Design review of the part shown in the three views and the two pictorial views. Dimensions are in mm from the part's minimum x, y and z. Coordinates: 2 decimals unless noted, no trailing zeros. Loops run counter-clockwise (first coordinate to the right, second up) from the corner with the lowest first, then second, coordinate; pieces in that order, holes last. Notation, with made-up numbers: (26, 75.25) -> (50, 75.25) arc R22 cw to (50, 89.25) -> close; hole circle Ø9 at (-34, 84). An arc over 180 degrees is marked (long way). Use a Markdown table: item, result. Add a question column.
Q1. For probe 1 along Y at (x, z) = (13.5, 5.75) (3 decimals); probe 2 along Z at (x, y) = (6, 11); probe 3 along X at (y, z) = (10.25, 6.5), list the stretches that pass through material, from the lowest coordinate up.
Q2. Clearance check with flat-ended pins moving along their axes: pin 1 Ø4 at (x, z) = (19.5, 2) entering from +Y; pin 2 Ø1 at (y, z) = (20.5, 1) entering from -X; pin 3 Ø1.2 at (x, y) = (13, 12.5) entering from +Z. State where each tip first meets the part, or that it passes through.
Q3. Take a section at C-C on z = 5. Write out the cut boundary in (x, y) (3 decimals), plus the area to 3 significant figures.
Q4. Draft analysis for pull direction X (two halves, no side actions). For the marked faces 1, 2 and 3, state which applies: pulls with the +X half, pulls with the -X half, needs draft (parallel to the pull), parting line crosses it, or undercut.
Q5. Take a section at A-A on x = 13.5. Write out the cut boundary in (y, z) (3 decimals).
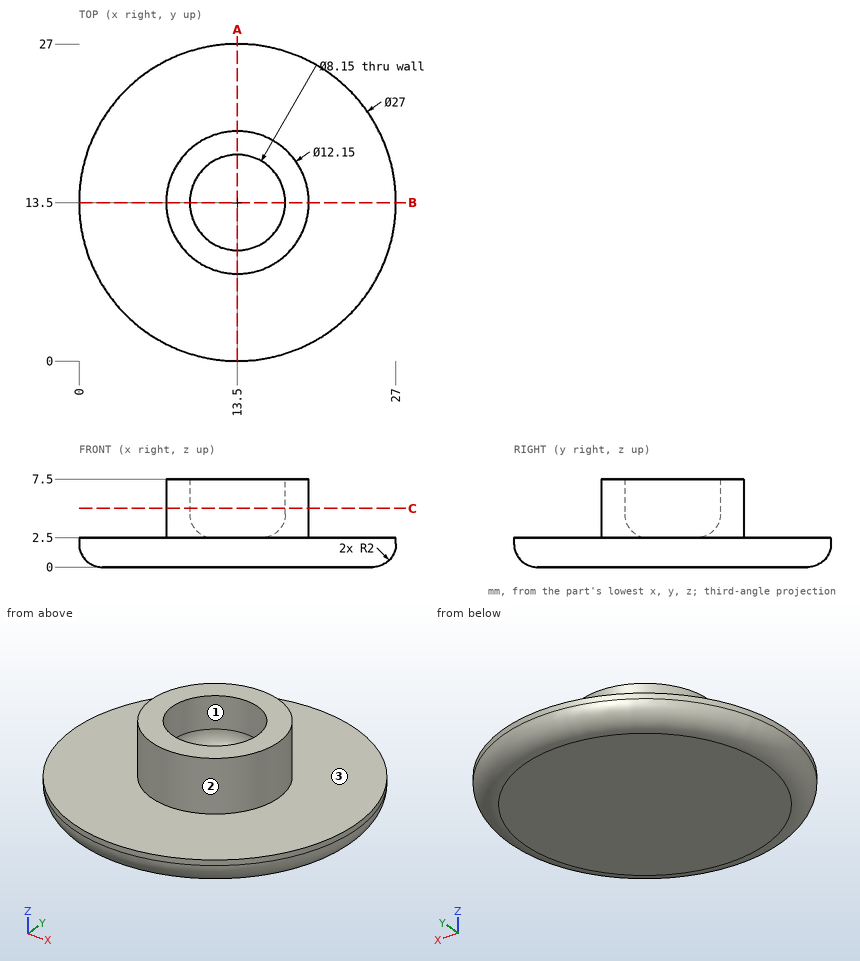
Answer list:
| question | item | result |
|---|---|---|
| 1 | probe 1 | 7.425 to 9.425, 17.575 to 19.575 |
| 1 | probe 2 | 0 to 2.5 |
| 1 | probe 3 | 8.37 to 11.04, 15.96 to 18.63 |
| 2 | pin 1 | y = 26.39 |
| 2 | pin 2 | x = 1.87 |
| 2 | pin 3 | z = 2.5 |
| 3 | outline | circle Ø12.15 at (13.5, 13.5); hole circle Ø8.15 at (13.5, 13.5) |
| 3 | area | 63.8 mm² |
| 4 | face 1 | undercut |
| 4 | face 2 | parting line crosses it |
| 4 | face 3 | needs draft |
| 5 | outline | (0, 2) arc R2 ccw to (2, 0) -> (25, 0) arc R2 ccw to (27, 2) -> (27, 2.5) -> (19.575, 2.5) -> (19.575, 7.5) -> (17.575, 7.5) -> (17.575, 4.5) arc R2 cw to (15.575, 2.5) -> (11.425, 2.5) arc R2 cw to (9.425, 4.5) -> (9.425, 7.5) -> (7.425, 7.5) -> (7.425, 2.5) -> (0, 2.5) -> close |
